```python
from build123d import *

# Parameters (mm, degrees)
SKETCH_1_R          = 37.5
EXTRUDE_1_DEPTH     = 50
SKETCH_2_R          = 32.5
CUT_EXTRUDE_1_DEPTH = 40
SKETCH_3_R          = 17.5
EXTRUDE_2_DEPTH     = 15
SKETCH_4_R          = 14.5
CUT_EXTRUDE_3_DEPTH = 84.889808678
SKETCH_6_R          = 3.5
CUT_EXTRUDE_4_DEPTH = 73.886898686
SKETCH_8_R          = 3.25
CUT_EXTRUDE_5_DEPTH = 73.886898686


with BuildPart() as part:
    # 草图1 → 凸台-拉伸1 (new body)
    with BuildSketch(Plane(origin=(0, 0, 0), x_dir=(1, 0, 0), z_dir=(0, 1, 0))):
        with Locations(Location((0, 0, 0), (0, 0, 270))):
            Circle(SKETCH_1_R)
    extrude(amount=EXTRUDE_1_DEPTH)

    # 草图2 → 切除-拉伸1 (cut)
    with BuildSketch(Plane(origin=(0, 50, 0), x_dir=(1, 0, 0), z_dir=(0, 1, 0))):
        with Locations(Location((0, 0, 0), (0, 0, 270))):
            Circle(SKETCH_2_R)
    extrude(amount=-CUT_EXTRUDE_1_DEPTH, mode=Mode.SUBTRACT)

    # 草图3 → 凸台-拉伸2 (add)
    with BuildSketch(Plane.XZ):
        with Locations(Location((0, 0, 0), (0, 0, 270))):
            Circle(SKETCH_3_R)
    extrude(amount=EXTRUDE_2_DEPTH)

    # 草图4 → 切除-拉伸3 (cut, through all)
    with BuildSketch(Plane(origin=(0, -15, 0), x_dir=(-1, 0, 0), z_dir=(0, -1, 0))):
        with Locations(Location((0, 0, 0), (0, 0, 90))):
            Circle(SKETCH_4_R)
    extrude(amount=-CUT_EXTRUDE_3_DEPTH, mode=Mode.SUBTRACT)

    # 草图6 → 切除-拉伸4 (cut, through all)
    with BuildSketch(Plane(origin=(0, 0, 0), x_dir=(-1, 0, 0), z_dir=(0, -1, 0))):
        with Locations(Location((-25.978212638, 0.984986916, 0), (0, 0, 90))):
            Circle(SKETCH_6_R)
    extrude(amount=-CUT_EXTRUDE_4_DEPTH, mode=Mode.SUBTRACT)

    # 草图8 → 切除-拉伸5 (cut, through all)
    with BuildSketch(Plane.XZ):
        with Locations(Location((-27.352744553, 0, 0), (0, 0, 270))):
            Circle(SKETCH_8_R)
    extrude(amount=-CUT_EXTRUDE_5_DEPTH, mode=Mode.SUBTRACT)


solid = part.part
```
CAD build for the part. Positions are in the model's coordinates, mm. A direction names the side the tool comes from. Round coordinates to 2 decimals unless told otherwise and drop trailing zeros. Loops run counter-clockwise (first coordinate to the right, second up) from the corner with the lowest first, then second, coordinate; pieces in that order, holes last. Notation, with made-up numbers: M 74.25,44 L 115.25,44 A20 cw 115.25,77 Z; hole C 55,46 d6. An arc over 180 degrees is marked long. Return JSON: item names as keys, results as strings. Group by question number.
(1) Saw through at A-A, the plane x = 0. List the corners of the cut face in (y, z), and give its area (3 significant figures).
(2) Saw through at C-C, the plane x = 8.5. List the corners of the cut face in (y, z).
(3) Saw through at B-B, the plane z = 0. List the corners of the cut face in (x, y), and give its area (3 significant figures).
(4) Tool access for faces 1 (the flat face through (-16, 0, 8)), 2 (the flat face through (31, 50, -11)), 3 (the flat face through (-7, 10, 14)): list every direction of +Z, -Z, +X, -X, +Y, -Y with a clear straight run to the whole face (end or side of a thin tool).
(5) Saw through at D-D, the plane y = 15.5. List the corners of the cut face in (x, z), and give its area (3 significant figures).
(6) Drop flat-ended pins along their axis: P1, Ø7.5, axis at x = -27.35, z = 0, coming from the -Y side; P2, Ø6, axis at x = 18.5, z = 3.5, coming from the -Y side; P3, Ø3, axis at y = 36.5, z = 18, coming from the -X side; P4, Ø10, axis at x = -17, y = 14, coming from the +Z side. Give the stop position or say it passes through.
(7) Mould opens along Z. For faces 4 (the flat face through (13, -15, 7)), 5 (the cylindrical face through (9.76, 30.28, 31)), 6 (the cylindrical face through (-22.818, 24.65, -29.759)) say: +Z half, -Z half, draft (parallel to the pull), parting line (faces both ways), or undercut.
(8) Wall check: probe 1 along X at (y, z) = (36, 0); probe 2 along Y at (x, z) = (10, 15); probe 3 along Y at (x, z) = (13, -32.5). Give the ranges that are in metal, low to high. Write a range as [from, to].
Answer list:
{
 "1": {"outline": "M -15,-17.5 L 0,-17.5 L 0,-37.5 L 50,-37.5 L 50,-32.5 L 10,-32.5 L 10,-14.5 L -15,-14.5 Z; M -15,14.5 L 10,14.5 L 10,32.5 L 50,32.5 L 50,37.5 L 0,37.5 L 0,17.5 L -15,17.5 Z", "area": "950 mm2"},
 "2": {"outline": "M -15,-15.3 L 0,-15.3 L 0,-36.52 L 50,-36.52 L 50,-31.37 L 10,-31.37 L 10,-11.75 L -15,-11.75 Z; M -15,11.75 L 10,11.75 L 10,31.37 L 50,31.37 L 50,36.52 L 0,36.52 L 0,15.3 L -15,15.3 Z"},
 "3": {"outline": "M -37.5,0 L -30.6,0 L -30.6,10 L -32.5,10 L -32.5,50 L -37.5,50 Z; M -24.1,0 L -17.5,0 L -17.5,-15 L -14.5,-15 L -14.5,10 L -24.1,10 Z; M 14.5,-15 L 17.5,-15 L 17.5,0 L 22.62,0 L 22.62,10 L 14.5,10 Z; M 29.34,0 L 37.5,0 L 37.5,50 L 32.5,50 L 32.5,10 L 29.34,10 Z", "area": "818 mm2"},
 "4": {"face 1": "-Y", "face 2": "+Z, -Z, +X, -X, +Y", "face 3": "+Y"},
 "5": {"outline": "C 0,0 d75; hole C 0,0 d65", "area": "1,100 mm2"},
 "6": {"P1": "y = 0", "P2": "y = -15", "P3": "x = -33.67", "P4": "z = 35.53"},
 "7": {"face 4": "draft", "face 5": "undercut", "face 6": "parting line"},
 "8": {"probe 1": "[-37.5, -32.5], [32.5, 37.5]", "probe 2": "[0, 10]", "probe 3": "[0, 50]"}
}
